Build history of the part. All positions in model axes, mm. Face numbers are marked on the shaded views. A direction names the side the tool comes from. Coordinates: 2 decimals unless noted, no trailing zeros. Loops run counter-clockwise (first coordinate to the right, second up) from the corner with the lowest first, then second, coordinate; pieces in that order, holes last.
Item 1: Cut at D-D (x = -14). List the corners of the cut face in (y, z) (3 decimals), and give its area (3 significant figures).
Item 2: Drill centre lines: line 1 along Y through (x, z) = (-24, 10); line 2 along Y through (x, z) = (-26, 6.5) (3 decimals); line 3 along Y through (x, z) = (17, 5.5) (3 decimals). Where is each one in solid material? Low to high.
Item 3: Mould opens along Y. For the marked faces 3, 4 and 5 say: released by +Y, released by -Y, zero draft, split by the parting line, or undercut.
Item 4: Flat gauge pin, fed straight in: pin 1 (5 mm diameter, centred on x = 23, y = 13.5, fed in from -Z). Where does the tip first touch, or does it go through?
Item 5: Cut at B-B (z = 13.75). List the corners of the cut face in (x, y), and give its area (3 significant figures).
Item 6: Cut at A-A (z = 5.25). List the corners of the cut face in (x, y) (3 decimals).
Item 7: Cut at C-C (x = 7). List the corners of the cut face in (y, z) (3 decimals), and give its area (3 significant figures).
Item 8: 3-axis set-ups, long thin cutter, end or side, ignore diameter. For the marked faces 1 and 2: which of +Z, -Z, +X, -X, +Y, -Y reach the whole face in a straight line?
from build123d import *

# Parameters (mm, degrees)
SKETCH_W        = 80
SKETCH_H        = 100
PAD_DEPTH       = 20
SKETCH001_W     = 100
SKETCH001_H     = 70.25
POCKET_DEPTH    = 8
POCKET001_DEPTH = 20.001
POCKET002_DEPTH = 20.001
FILLET_R        = 14
SKETCH004_W     = 200
SKETCH004_H     = 6
POCKET003_DEPTH = 0.5


with BuildPart() as part:
    # Sketch → Pad (new body)
    with BuildSketch(Plane.XY):
        Rectangle(SKETCH_W, SKETCH_H)
    extrude(amount=PAD_DEPTH)

    # Sketch001 → Pocket (cut)
    with BuildSketch(Plane(origin=(0, 0, 0), x_dir=(1, 0, 0), z_dir=(0, 0, -1))):
        Rectangle(SKETCH001_W, SKETCH001_H)
    extrude(amount=-POCKET_DEPTH, mode=Mode.SUBTRACT)

    # Sketch002 → Pocket001 (cut, through all)
    with BuildSketch(Plane(origin=(0, 0, 0), x_dir=(1, 0, 0), z_dir=(0, 0, -1))):
        Polygon((-32, 46), (-12, 46), (-9, 43), (-12, 40), (-32, 40), (-35, 43), align=None)
        Polygon((0, 45), (-2.828427, 42.171573), (0, 39.343146), (2.828427, 42.171573), align=None)
    extrude(amount=-POCKET001_DEPTH, mode=Mode.SUBTRACT)

    # Sketch003 → Pocket002 (cut, through all)
    with BuildSketch(Plane.XY.offset(20)):
        Polygon((-21.213203, 0), (0, 21.213203), (21.213203, 0), (0, -21.213203), align=None)
    extrude(amount=-POCKET002_DEPTH, mode=Mode.SUBTRACT)

    # Fillet
    fillet_edges = [part.edges().sort_by_distance(p)[0] for p in [
        (0, 21.213203, 14),
        (-21.213203, 0, 14),
        (0, -21.213203, 14),
    ]]
    fillet(fillet_edges, radius=FILLET_R)

    # Sketch004 → Pocket003 (cut)
    with BuildSketch(Plane(origin=(0, -35.125, 0), x_dir=(-1, 0, 0), z_dir=(0, 1, 0))):
        with Locations((0, 5)):
            Rectangle(SKETCH004_W, SKETCH004_H)
    extrude(amount=-POCKET003_DEPTH, mode=Mode.SUBTRACT)


solid = part.part
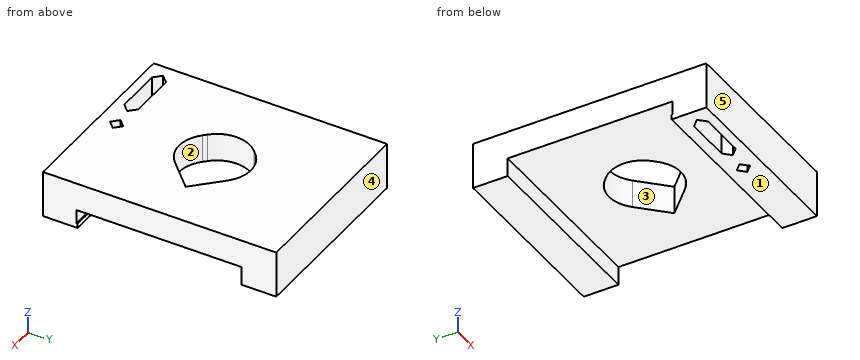
Filled sheet:
1. outline: (-50, 0) - (-46, 0) - (-46, 20) - (-50, 20) - close; (-40, 0) - (-35.125, 0) - (-35.125, 2) - (-35.625, 2) - (-35.625, 8) - (-6.132, 8) - (-6.132, 20) - (-40, 20) - close; (6.132, 8) - (35.125, 8) - (35.125, 0) - (50, 0) - (50, 20) - (6.132, 20) - close
1. area: 1,170 mm2
2. line 1: y = -50 to -46, -40 to 50
2. line 2: y = -50 to -46, -40 to -35.625, 35.125 to 50
2. line 3: y = -50 to -35.625, 35.125 to 50
3. face 3: undercut
3. face 4: released by +Y
3. face 5: released by -Y
4. pin 1: stops at z = 8
5. outline: (-40, -50) - (40, -50) - (40, 50) - (-40, 50) - close; hole (-35, -43) - (-32, -46) - (-12, -46) - (-9, -43) - (-12, -40) - (-32, -40) - close; hole (-11.31, -9.9) - (-9.9, -11.31) arc R14 ccw to (9.9, -11.31) - (21.21, 0) - (9.9, 11.31) arc R14 ccw to (-9.9, 11.31) - (-11.31, 9.9) arc R14 ccw to start; hole (-2.83, -42.17) - (0, -45) - (2.83, -42.17) - (0, -39.34) - close
5. area: 7,070 mm2
6. outline: (-40, -50) - (40, -50) - (40, -35.625) - (-40, -35.625) - close; (-40, 35.125) - (40, 35.125) - (40, 50) - (-40, 50) - close; hole (-35, -43) - (-32, -46) - (-12, -46) - (-9, -43) - (-12, -40) - (-32, -40) - close; hole (-2.828, -42.172) - (0, -45) - (2.828, -42.172) - (0, -39.343) - close
7. outline: (-50, 0) - (-35.125, 0) - (-35.125, 2) - (-35.625, 2) - (-35.625, 8) - (-13.539, 8) - (-13.539, 20) - (-50, 20) - close; (13.539, 8) - (35.125, 8) - (35.125, 0) - (50, 0) - (50, 20) - (13.539, 20) - close
7. area: 1,110 mm2
8. face 1: -Z, +X, -X, +Y, -Y
8. face 2: +Z, -Z
